Geometry check sheet. Reference: the model listing, model coordinates, mm. A direction names the side the tool comes from. Give positions to 0.01 mm unless a question says otherwise; leave off trailing zeros. Loops run counter-clockwise (first coordinate to the right, second up) from the corner with the lowest first, then second, coordinate; pieces in that order, holes last.
```python
from build123d import *

# Parameters (mm, degrees)
F0_R     = 10.5
F0_R_2   = 9.7
F0_R_3   = 9.5
F0_R_4   = 8.5
F2_DEPTH = 115
F3_DEPTH = 20
F4_DEPTH = 12.5


with BuildPart() as f2:
    # F0 (on Top) → F2 (new body)
    with BuildSketch(Plane.XY):
        Circle(F0_R)
        Circle(F0_R_2, mode=Mode.SUBTRACT)
        Circle(F0_R_2)
        Circle(F0_R_3, mode=Mode.SUBTRACT)
        Circle(F0_R_3)
        Circle(F0_R_4, mode=Mode.SUBTRACT)
    extrude(amount=F2_DEPTH)

    # F0 (on Top) → F3 (join)
    with BuildSketch(Plane.XY):
        Circle(F0_R)
        Circle(F0_R_2, mode=Mode.SUBTRACT)
    extrude(amount=-F3_DEPTH)

    # F1 (on Front) → F4 (cut, symmetric)
    with BuildSketch(Plane.XZ):
        with BuildLine():
            Line((-0.0001868698, 87.999952428), (-0.0001868698, 81.999952428))
            ThreePointArc((-0.0001868698, 81.999952428), (2.1211334738, 82.8786320845), (2.9998131302, 84.999952428))
            ThreePointArc((2.9998131302, 84.999952428), (2.1211334738, 87.1212727716), (-0.0001868698, 87.999952428))
        make_face()
        with BuildLine():
            ThreePointArc((-0.0001868698, 87.999952428), (-3.0001868698, 84.999952428), (-0.0001868698, 81.999952428))
            Line((-0.0001868698, 81.999952428), (-0.0001868698, 87.999952428))
        make_face()
        with BuildLine():
            ThreePointArc((-0.0001868698, 97.999952428), (-3.0001868698, 94.999952428), (-0.0001868698, 91.999952428))
            Line((-0.0001868698, 91.999952428), (-0.0001868698, 97.999952428))
        make_face()
        with BuildLine():
            Line((-0.0001868698, 97.999952428), (-0.0001868698, 91.999952428))
            ThreePointArc((-0.0001868698, 91.999952428), (2.1211334738, 92.8786320845), (2.9998131302, 94.999952428))
            ThreePointArc((2.9998131302, 94.999952428), (2.1211334738, 97.1212727716), (-0.0001868698, 97.999952428))
        make_face()
        with BuildLine():
            ThreePointArc((2.9998131302, 104.999952428), (2.1211334738, 107.1212727716), (-0.0001868698, 107.999952428))
            Line((-0.0001868698, 107.999952428), (-0.0001868698, 101.999952428))
            ThreePointArc((-0.0001868698, 101.999952428), (2.1211334738, 102.8786320845), (2.9998131302, 104.999952428))
        make_face()
        with BuildLine():
            Line((-0.0001868698, 101.999952428), (-0.0001868698, 107.999952428))
            ThreePointArc((-0.0001868698, 107.999952428), (-3.0001868698, 104.999952428), (-0.0001868698, 101.999952428))
        make_face()
    extrude(amount=F4_DEPTH, both=True, mode=Mode.SUBTRACT)


solid = f2.part
```
1) Depth check by flat-ended pin: P1, Ø5, axis at y = -4, z = -5.5, coming from the -X side; P2, Ø5, axis at y = -3.5, z = 75.5, coming from the +X side; P3, Ø1.5, axis at y = 2, z = -1, coming from the +X side. Enter the tip coordinate at first touch or a pass-through.
2) Mould release check, pull along Y, two halves, no side actions. Record for faces 3 (the cylindrical face through (10, 3.2, 48.4)), 4 (the flat face through (0, -9, 0)), 5 (the flat face through (9, 0, 115)): +Y half, -Y half, draft (parallel to the pull), parting line (faces both ways), or undercut.
3) Scan lines: line 1 along X through (y, z) = (-0.5, 8.5); line 2 along Y through (x, z) = (0.25, -13); line 3 along Z through (x, y) = (0.5, 8.75). Record each from-to range of solid material in increasing order.
4) Sectioned sample at B-B on x = 6. Enter the section's corners in (y, z).
5) Tool access check on faces 1 (the cylindrical face through (-2.662, -9.211, 83.616)), 2 (the cylindrical face through (9.252, 2.914, -9.86)). Record the directions out of +Z, -Z, +X, -X, +Y, -Y that give a thin tool (end or side, any length) a straight path to the whole face; none if there is none.
6) Sectioned sample at C-C on z = 62. Enter the section's corners in (x, y).
7) Sectioned sample at A-A on y = 0. Enter the section's corners in (x, z).
Determined:
1. P1: stops at x = -10.39
1. P2: stops at x = 10.45
1. P3: stops at x = 10.43
2. face 3: parting line
2. face 4: undercut
2. face 5: draft
3. line 1: x = -10.49 to -8.49, 8.49 to 10.49
3. line 2: y = -10.5 to -9.7, 9.7 to 10.5
3. line 3: z = 0 to 82.04, 87.96 to 92.04, 97.96 to 102.04, 107.96 to 115
4. outline: (-8.62, -20) - (-7.62, -20) - (-7.62, 0) - (-6.02, 0) - (-6.02, 115) - (-8.62, 115) - close; (6.02, 0) - (7.62, 0) - (7.62, -20) - (8.62, -20) - (8.62, 115) - (6.02, 115) - close
5. face 1: +Y, -Y
5. face 2: -Z
6. outline: circle Ø21 at (0, 0); hole circle Ø17 at (0, 0)
7. outline: (-10.5, -20) - (-9.7, -20) - (-9.7, 0) - (-8.5, 0) - (-8.5, 115) - (-10.5, 115) - close; (8.5, 0) - (9.7, 0) - (9.7, -20) - (10.5, -20) - (10.5, 115) - (8.5, 115) - close
